```python
from build123d import *

# Parameters (mm, degrees)
SKETCH1_W           = 127
SKETCH1_H           = 76.2
BOSS_EXTRUDE1_DEPTH = 38.1
SKETCH2_R           = 6.35
CUT_EXTRUDE2_DEPTH  = 84.279469259
SKETCH3_W           = 38.1
SKETCH3_H           = 76.2
CUT_EXTRUDE3_DEPTH  = 25.4
FILLET1_R           = 17.78
CHAMFER1_SIZE       = 3.175
SHELL1_T            = -2.54
FILLET2_R           = 2.54


with BuildPart() as part:
    # Sketch1 → Boss-Extrude1 (new body)
    with BuildSketch(Plane(origin=(0, 0, 0), x_dir=(1, 0, 0), z_dir=(0, 1, 0))):
        Rectangle(SKETCH1_W, SKETCH1_H)
    extrude(amount=BOSS_EXTRUDE1_DEPTH)

    # Sketch2 → Cut-Extrude2 (cut, through all)
    with BuildSketch(Plane(origin=(0, 38.1, 0), x_dir=(1, 0, 0), z_dir=(0, 1, 0))):
        with Locations(Location((-44.45, 19.05, 0), (0, 0, 270))):
            Circle(SKETCH2_R)
        with Locations(Location((44.45, 19.05, 0), (0, 0, 270))):
            Circle(SKETCH2_R)
        with Locations(Location((44.45, -19.05, 0), (0, 0, 270))):
            Circle(SKETCH2_R)
        with Locations(Location((-44.45, -19.05, 0), (0, 0, 270))):
            Circle(SKETCH2_R)
    extrude(amount=-CUT_EXTRUDE2_DEPTH, mode=Mode.SUBTRACT)

    # Sketch3 → Cut-Extrude3 (cut)
    with BuildSketch(Plane(origin=(0, 38.1, 0), x_dir=(1, 0, 0), z_dir=(0, 1, 0))):
        Rectangle(SKETCH3_W, SKETCH3_H)
    extrude(amount=-CUT_EXTRUDE3_DEPTH, mode=Mode.SUBTRACT)

    # Fillet1
    fillet1_edges = [part.edges().sort_by_distance(p)[0] for p in [
        (63.5, 19.05, 38.1),
        (-63.5, 19.05, 38.1),
        (-63.5, 19.05, -38.1),
        (63.5, 19.05, -38.1),
    ]]
    fillet(fillet1_edges, radius=FILLET1_R)

    # Chamfer1
    chamfer1_edges = [part.edges().sort_by_distance(p)[0] for p in [
        (-44.45, 38.1, 12.7),
        (44.45, 38.1, 12.7),
        (44.45, 38.1, -25.4),
        (-44.45, 38.1, -25.4),
    ]]
    chamfer(chamfer1_edges, length=CHAMFER1_SIZE)

    # Shell1
    shell1_openings = [part.faces().sort_by_distance(p)[0] for p in [
        (0, 0, 0),
    ]]
    offset(amount=SHELL1_T, openings=shell1_openings, kind=Kind.INTERSECTION)

    # Fillet2
    fillet2_edges = [part.edges().sort_by_distance(p)[0] for p in [
        (-32.385, 38.1, -38.1),
        (32.385, 38.1, 38.1),
        (19.05, 12.7, 0),
        (19.05, 25.4, -38.1),
        (0, 12.7, 38.1),
        (19.05, 25.4, 38.1),
        (-19.05, 12.7, 0),
        (-19.05, 25.4, 38.1),
        (0, 12.7, -38.1),
        (-19.05, 25.4, -38.1),
        (19.05, 38.1, 0),
        (-19.05, 38.1, 0),
        (-63.5, 38.1, 0),
        (32.385, 38.1, -38.1),
        (-32.385, 38.1, 38.1),
        (-58.292358569, 38.1, 32.892358569),
        (-58.292358569, 38.1, -32.892358569),
        (63.5, 38.1, 0),
        (58.292358569, 38.1, 32.892358569),
        (58.292358569, 38.1, -32.892358569),
    ]]
    fillet(fillet2_edges, radius=FILLET2_R)


solid = part.part
```
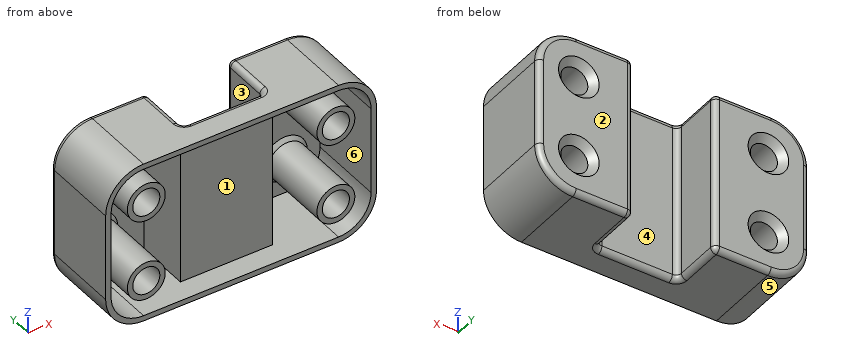
Model file for the job. Use its own axes, mm. Face numbers are marked on the shaded views. A direction names the side the tool comes from. Coordinates: 2 decimals unless noted, no trailing zeros. Write each loop counter-clockwise with the first axis right and the second up, starting at its lowest first coordinate (ties: lowest second). Pieces come first, ordered by that corner, then holes. Notation, with made-up numbers: (-1, -3.5) - (37, -3.5) arc R31 cw to (37, 32.5) - close; hole circle Ø2 at (2.25, 66.25). An arc over 180 degrees is marked (long way). One line per item, written item: value. Start each with the question number.
1. Slice it at A-A (x = -44.45). Count the separate pieces of the cut face and the enclosed holes in it, plus the area to 3 significant figures.
2. Slice it at C-C (x = 7). Write the cut outline in (y, z), plus the area to 3 significant figures.
3. Flat gauge pins, fed straight in: pin 1 (7.5 mm diameter, centred on x = -44.45, z = -19.05, fed in from -Y); pin 2 (10 mm diameter, centred on x = 6.5, z = 7, fed in from +Y); pin 3 (2 mm diameter, centred on y = 26.5, z = 24, fed in from -X); pin 4 (10 mm diameter, centred on y = 8.5, z = -27, fed in from +X). Where does each tip first touch, or does it go through?
4. Tool access for the marked faces 1, 2 and 3: list every direction of +Z, -Z, +X, -X, +Y, -Y with a clear straight run to the whole face (end or side of a thin tool).
5. Mould opens along Z. For the marked faces 4, 5 and 6 say: released by +Z, released by -Z, zero draft, split by the parting line, or undercut.
6. Probe line 1 (Z direction, x = -44, y = 14); line 2 (X direction, y = 25, z = 8); line 3 (X direction, y = 10, z = 19). List the from-to ranges inside material, lowest first. Write a range as from..to.
Answers below:
1. separate pieces: 3
1. enclosed holes: 0
1. area: 654 mm^2
2. outline: (0, -38.1) - (10.16, -38.1) arc R2.54 ccw to (12.7, -35.56) - (12.7, 35.56) arc R2.54 ccw to (10.16, 38.1) - (0, 38.1) - (0, 35.56) - (10.16, 35.56) - (10.16, -35.56) - (0, -35.56) - close
2. area: 242 mm^2
3. pin 1: passes through
3. pin 2: stops at y = 12.7
3. pin 3: stops at x = -63.3
3. pin 4: stops at x = 63.42
4. face 1: -Y
4. face 2: +Z, -Z, +X, -X, +Y
4. face 3: +Z, -Z, +Y
5. face 4: zero draft
5. face 5: released by -Z
5. face 6: undercut
6. line 1: z = -38.1..-35.56, -27.93..-25.38, -12.72..-10.17, 10.17..12.72, 25.38..27.93, 35.56..38.1
6. line 2: x = -63.5..-60.96, -21.59..-19.05, 19.05..21.59, 60.96..63.5
6. line 3: x = -63.5..-60.96, -53.34..-50.8, -38.1..-35.56, 35.56..38.1, 50.8..53.34, 60.96..63.5
